Geometry check sheet. Reference: the model listing, model coordinates, mm. A direction names the side the tool comes from. Give positions to 0.01 mm unless a question says otherwise; leave off trailing zeros. Loops run counter-clockwise (first coordinate to the right, second up) from the corner with the lowest first, then second, coordinate; pieces in that order, holes last. Notation, with made-up numbers: (42, -31.75) -> (63, -31.75) arc R25 cw to (63, 7.25) -> close; hole circle Ø11 at (-7.5, 1). An arc over 180 degrees is marked (long way). Write each question's results on one line, items separated by ' | '. Start each with the question number.
1) Scan lines: line 1 (X direction, y = 5.75, z = 26); line 2 (X direction, y = 3, z = 46) (3 decimals); line 3 (X direction, y = 2.75, z = 40). Record each from-to range of solid material in increasing order. Write a range as from..to.
2) Set-up check for faces 1 (the face through (5.3, 2.96, 23.35)), 2 (the face through (0, 3, 50)), 3 (the face through (15.72, 2.52, 45.69)): record each of +Z, -Z, +X, -X, +Y, -Y from which the full face is reachable in a straight line by a thin tool's end or side.
3) Sectioned sample at A-A on x = -9.5. Record the cut outline in (y, z).
4) Draft check along Y on faces 4 (the face through (-5.78, 3.15, 40.88)), 5 (the face through (-16.67, 2.92, 40.88)), 6 (the face through (0, 6, 13)), 7 (the face through (-0.046, 3.042, 2.087)). Enter one of: pulls with the +Y half, pulls with the -Y half, needs draft (parallel to the pull), parting line crosses it, or undercut.
5) Depth check by flat-ended pin: pin 1 (1.5 mm diameter, centred on x = -16, z = 13, fed in from -Y); pin 2 (2.5 mm diameter, centred on x = 3, y = 3, fed in from -Z); pin 3 (1.8 mm diameter, centred on y = 3.5, z = -5, fed in from -X); pin 4 (1.8 mm diameter, centred on y = 2.5, z = -16.5, fed in from +X). Enter the tip coordinate at first touch or a pass-through.
6) Sectioned sample at B-B on x = 9. Record the cut outline in (y, z), then the cut area to 3 significant figures.
```python
from build123d import *

# Parameters (mm, degrees)
EXTRUDE_1_DEPTH     = 6
CUT_EXTRUDE_1_DEPTH = 56.156595254
CUT_EXTRUDE_2_REACH = 57.157
FILLET_18_R         = 2
M3X0_51_D           = 2.5
M3X0_51_DEPTH       = 8.5
M3X0_51_TIP         = 0.751075774


with BuildPart() as part:
    # Эскиз1 → Бобышка-Вытянуть1 (new body)
    with BuildSketch(Plane(origin=(0, 0, 0), x_dir=(1, 0, 0), z_dir=(0, 1, 0))):
        with BuildLine():
            Line((-22.5, 0), (-22.5, -50))
            Line((-22.5, -50), (22.5, -50))
            Line((22.5, -50), (22.5, 0))
            ThreePointArc((22.5, 0), (0, 22.5), (-22.5, 0))
        make_face()
    extrude(amount=EXTRUDE_1_DEPTH)

    # Эскиз2 → Вырез-Вытянуть1 (cut, through all)
    with BuildSketch(Plane(origin=(0, 6, 0), x_dir=(1, 0, 0), z_dir=(0, 1, 0))):
        with BuildLine():
            Line((-10.274368671, 12.374368671), (-10.274368671, -40))
            ThreePointArc((-10.274368671, -40), (-12.374368671, -42.1), (-14.474368671, -40))
            Line((-14.474368671, -40), (-14.474368671, 12.374368671))
            ThreePointArc((-14.474368671, 12.374368671), (-12.374368671, 14.474368671), (-10.274368671, 12.374368671))
        make_face()
        with BuildLine():
            Line((10.274368671, 12.374368671), (10.274368671, -40))
            ThreePointArc((10.274368671, -40), (12.374368671, -42.1), (14.474368671, -40))
            Line((14.474368671, -40), (14.474368671, 12.374368671))
            ThreePointArc((14.474368671, 12.374368671), (12.374368671, 14.474368671), (10.274368671, 12.374368671))
        make_face()
    extrude(amount=-CUT_EXTRUDE_1_DEPTH, mode=Mode.SUBTRACT)

    # Эскиз11 → Вырез-Вытянуть2 (cut, up to next)
    with BuildSketch(Plane(origin=(0, 6, 0), x_dir=(1, 0, 0), z_dir=(0, 1, 0)), mode=Mode.PRIVATE) as cut_extrude_2_sk1:
        with BuildLine():
            Line((6.274368671, 18.5), (-6.274368671, 11.254983118))
            Line((-6.274368671, 11.254983118), (-6.274368671, 18.5))
            ThreePointArc((-6.274368671, 18.5), (0, 19.535037809), (6.274368671, 18.5))
        make_face()
    cut_extrude_2_tool1 = extrude(cut_extrude_2_sk1.sketch, amount=-CUT_EXTRUDE_2_REACH, mode=Mode.PRIVATE) & part.part
    # Эскиз11 → Вырез-Вытянуть2 (cut, up to next)
    with BuildSketch(Plane(origin=(0, 6, 0), x_dir=(1, 0, 0), z_dir=(0, 1, 0)), mode=Mode.PRIVATE) as cut_extrude_2_sk2:
        Polygon((6.274368671, 13.627163728), (-6.274368671, 6.382146846), (6.274368671, -0.862870036), align=None)
    cut_extrude_2_tool2 = extrude(cut_extrude_2_sk2.sketch, amount=-CUT_EXTRUDE_2_REACH, mode=Mode.PRIVATE) & part.part
    # Эскиз11 → Вырез-Вытянуть2 (cut, up to next)
    with BuildSketch(Plane(origin=(0, 6, 0), x_dir=(1, 0, 0), z_dir=(0, 1, 0)), mode=Mode.PRIVATE) as cut_extrude_2_sk3:
        Polygon((-6.274368671, 1.509310574), (6.274368671, -5.735706308), (-6.274368671, -12.98072319), align=None)
    cut_extrude_2_tool3 = extrude(cut_extrude_2_sk3.sketch, amount=-CUT_EXTRUDE_2_REACH, mode=Mode.PRIVATE) & part.part
    # Эскиз11 → Вырез-Вытянуть2 (cut, up to next)
    with BuildSketch(Plane(origin=(0, 6, 0), x_dir=(1, 0, 0), z_dir=(0, 1, 0)), mode=Mode.PRIVATE) as cut_extrude_2_sk4:
        Polygon((-6.274368671, -17.853559462), (6.274368671, -10.60854258), (6.274368671, -25.098576344), align=None)
    cut_extrude_2_tool4 = extrude(cut_extrude_2_sk4.sketch, amount=-CUT_EXTRUDE_2_REACH, mode=Mode.PRIVATE) & part.part
    # Эскиз11 → Вырез-Вытянуть2 (cut, up to next)
    with BuildSketch(Plane(origin=(0, 6, 0), x_dir=(1, 0, 0), z_dir=(0, 1, 0)), mode=Mode.PRIVATE) as cut_extrude_2_sk5:
        Polygon((-6.274368671, -22.726395734), (6.274368671, -29.971412616), (-6.274368671, -37.216429498), align=None)
    cut_extrude_2_tool5 = extrude(cut_extrude_2_sk5.sketch, amount=-CUT_EXTRUDE_2_REACH, mode=Mode.PRIVATE) & part.part
    # Эскиз11 → Вырез-Вытянуть2 (cut, up to next)
    with BuildSketch(Plane(origin=(0, 6, 0), x_dir=(1, 0, 0), z_dir=(0, 1, 0)), mode=Mode.PRIVATE) as cut_extrude_2_sk6:
        Polygon((-6.274368671, -42.08926577), (6.274368671, -34.844248888), (6.274368671, -42.08926577), align=None)
    cut_extrude_2_tool6 = extrude(cut_extrude_2_sk6.sketch, amount=-CUT_EXTRUDE_2_REACH, mode=Mode.PRIVATE) & part.part
    add(cut_extrude_2_tool1.solids().sort_by_distance((-1.755291, 6, -16.539864))[0], mode=Mode.SUBTRACT)
    add(cut_extrude_2_tool2.solids().sort_by_distance((2.091456, 6, -6.382147))[0], mode=Mode.SUBTRACT)
    add(cut_extrude_2_tool3.solids().sort_by_distance((-2.091456, 6, 5.735706))[0], mode=Mode.SUBTRACT)
    add(cut_extrude_2_tool4.solids().sort_by_distance((2.091456, 6, 17.853559))[0], mode=Mode.SUBTRACT)
    add(cut_extrude_2_tool5.solids().sort_by_distance((-2.091456, 6, 29.971413))[0], mode=Mode.SUBTRACT)
    add(cut_extrude_2_tool6.solids().sort_by_distance((2.091456, 6, 39.67426))[0], mode=Mode.SUBTRACT)

    # Скругление18
    fillet_18_edges = [part.edges().sort_by_distance(p)[0] for p in [
        (6.274368671, 3, -13.627163728),
        (6.274368671, 3, 0.862870036),
        (-6.274368671, 3, -6.382146846),
        (-6.274368671, 3, -18.5),
        (6.274368671, 3, -18.5),
        (-6.274368671, 3, -11.254983118),
        (-6.274368671, 3, 12.98072319),
        (-6.274368671, 3, -1.509310574),
        (6.274368671, 3, 5.735706308),
        (6.274368671, 3, 25.098576344),
        (-6.274368671, 3, 17.853559462),
        (6.274368671, 3, 10.60854258),
        (-6.274368671, 3, 37.216429498),
        (-6.274368671, 3, 22.726395734),
        (6.274368671, 3, 29.971412616),
        (6.274368671, 3, 42.08926577),
        (-6.274368671, 3, 42.08926577),
        (6.274368671, 3, 34.844248888),
    ]]
    fillet(fillet_18_edges, radius=FILLET_18_R)

    # Отверстие обработанное метчиком M3x0.51
    with Locations(Plane.XY.offset(50)):
        with Locations((-16.875, 3), (-5.625, 3), (5.625, 3), (16.875, 3)):
            Hole(M3X0_51_D / 2, depth=M3X0_51_DEPTH)
            with Locations((0, 0, -(M3X0_51_DEPTH + M3X0_51_TIP / 2))):  # 118° drill point
                Cone(0, M3X0_51_D / 2, M3X0_51_TIP, mode=Mode.SUBTRACT)


solid = part.part
```
Result:
1) line 1: -22.5..-14.47, -10.27..-6.27, -0.6..10.27, 14.47..22.5 | line 2: -22.5..-18.125, -15.625..-6.875, -4.375..4.375, 6.875..15.625, 18.125..22.5 | line 3: -22.5..-14.47, -10.27..-0.81, 6.27..10.27, 14.47..22.5
2) face 1: +Y, -Y | face 2: +Z, +X, -X, +Y, -Y | face 3: +Z
3) outline: (0, -20.4) -> (6, -20.4) -> (6, 50) -> (0, 50) -> close
4) face 4: undercut | face 5: undercut | face 6: pulls with the +Y half | face 7: needs draft
5) pin 1: y = 0 | pin 2: z = -22.43 | pin 3: x = -22.12 | pin 4: x = 16.21
6) outline: (0, -20.62) -> (6, -20.62) -> (6, 50) -> (0, 50) -> close | area: 424 mm^2
